from build123d import *

# Parameters (mm, degrees)
SKETCH_1_R          = 15
SKETCH_1_R_2        = 1.45
SKETCH_1_R_3        = 1.5
EXTRUDE_1_DEPTH     = 13
SKETCH_2_R          = 1.45
SKETCH_2_R_2        = 1.5
EXTRUDE_2_DEPTH     = 7
SKETCH_3_R          = 1.45
CUT_EXTRUDE_1_DEPTH = 38.5
SKETCH_4_R          = 1.45
CUT_EXTRUDE_2_DEPTH = 38.5
SKETCH_5_R          = 1.45
CUT_EXTRUDE_3_DEPTH = 31
SKETCH_8_R          = 1.5
CUT_EXTRUDE_6_DEPTH = 38.5
CHAMFER_1_SIZE      = 1.55


with BuildPart() as part:
    # 草图1 → 凸台-拉伸1 (new body)
    with BuildSketch(Plane(origin=(0, 0, 0), x_dir=(1, 0, 0), z_dir=(0, 1, 0))):
        Circle(SKETCH_1_R)
        with Locations((0, 12)):
            Circle(SKETCH_1_R_2, mode=Mode.SUBTRACT)
        with Locations((-10.392304845, -6)):
            Circle(SKETCH_1_R_2, mode=Mode.SUBTRACT)
        with Locations((10.392304845, -6)):
            Circle(SKETCH_1_R_2, mode=Mode.SUBTRACT)
        with Locations((-11.258330249, 6.5)):
            Circle(SKETCH_1_R_3, mode=Mode.SUBTRACT)
        with Locations((0, -13)):
            Circle(SKETCH_1_R_3, mode=Mode.SUBTRACT)
        with Locations((11.258330249, 6.5)):
            Circle(SKETCH_1_R_3, mode=Mode.SUBTRACT)
    extrude(amount=EXTRUDE_1_DEPTH)

    # 草图2 → 凸台-拉伸2 (add)
    with BuildSketch(Plane(origin=(0, 13, 0), x_dir=(1, 0, 0), z_dir=(0, 1, 0))):
        Polygon((0, 17.320508076), (-15, 8.660254038), (-15, -8.660254038), (0, -17.320508076), (15, -8.660254038), (15, 8.660254038), align=None)
        with Locations((0, 12)):
            Circle(SKETCH_2_R, mode=Mode.SUBTRACT)
        with Locations((-11.258330249, 6.5)):
            Circle(SKETCH_2_R_2, mode=Mode.SUBTRACT)
        with Locations((11.258330249, 6.5)):
            Circle(SKETCH_2_R_2, mode=Mode.SUBTRACT)
        with Locations((-10.392304845, -6)):
            Circle(SKETCH_2_R, mode=Mode.SUBTRACT)
        with Locations((0, -13)):
            Circle(SKETCH_2_R_2, mode=Mode.SUBTRACT)
        with Locations((10.392304845, -6)):
            Circle(SKETCH_2_R, mode=Mode.SUBTRACT)
    extrude(amount=-EXTRUDE_2_DEPTH)

    # 草图3 → 切除-拉伸1 (cut, through all)
    with BuildSketch(Plane(origin=(7.5, 0, 12.990381057), x_dir=(0.866025404, 0, -0.5), z_dir=(0.5, 0, 0.866025404))):
        with Locations((0, 9.5)):
            Circle(SKETCH_3_R)
    extrude(amount=-CUT_EXTRUDE_1_DEPTH, mode=Mode.SUBTRACT)

    # 草图4 → 切除-拉伸2 (cut, through all)
    with BuildSketch(Plane(origin=(-7.5, 0, 12.990381057), x_dir=(0.866025404, 0, 0.5), z_dir=(-0.5, 0, 0.866025404))):
        with Locations((0, 9.5)):
            Circle(SKETCH_4_R)
    extrude(amount=-CUT_EXTRUDE_2_DEPTH, mode=Mode.SUBTRACT)

    # 草图5 → 切除-拉伸3 (cut, through all)
    with BuildSketch(Plane.ZY.offset(15)):
        with Locations((0, 9.5)):
            Circle(SKETCH_5_R)
    extrude(amount=-CUT_EXTRUDE_3_DEPTH, mode=Mode.SUBTRACT)

    # 草图8 → 切除-拉伸6 (cut, through all)
    with BuildSketch(Plane(origin=(-7.5, 0, -12.990381057), x_dir=(-0.866025404, 0, 0.5), z_dir=(-0.5, 0, -0.866025404))):
        with Locations((0, 9.5)):
            Circle(SKETCH_8_R)
    extrude(amount=-CUT_EXTRUDE_6_DEPTH, mode=Mode.SUBTRACT)

    # 倒角1
    chamfer_1_edges = [part.edges().sort_by_distance(p)[0] for p in [
        (8.942304845, 13, 6),
        (-1.45, 13, -12),
        (-11.842304845, 13, 6),
    ]]
    chamfer(chamfer_1_edges, length=CHAMFER_1_SIZE)


solid = part.part
Design review of the part built by this model. Coordinates are the model's own, in mm. A direction names the side the tool comes from. Give positions to 0.01 mm unless a question says otherwise; leave off trailing zeros. Answer as a JSON object with one key per item and string values. Group by question number.
1) For line 1 along X through (y, z) = (3.5, 6); line 2 along Z through (x, y) = (0, 5); line 3 along Y through (x, z) = (6.5, 11), list the stretches that pass through material, from the lowest coordinate up.
2) We need section A-A (y = 8.5). Count the separate pieces of the cut face and the enclosed holes in it, and give its area (3 significant figures).
3) Tool access review of faces 1 (the face through (0, 6, 15.5)), 2 (the face through (13, 6, 8)), 3 (the face through (7.59, 9.56, -1.45)): name each direction out of +Z, -Z, +X, -X, +Y, -Y from which nothing blocks a thin tool from reaching the whole face with its end or side.
4) Clearance check with flat-ended pins moving along their axes: pin 1 Ø4 at (x, z) = (-11.26, -6.5) entering from -Y; pin 2 Ø1 at (y, z) = (8.5, 10.5) entering from -X; pin 3 Ø5 at (x, y) = (8.5, 1.5) entering from +Z; pin 4 Ø1.5 at (x, z) = (10.5, 7) entering from +Y. State where each tip first meets the part, or that it passes through.
5) Mouldability with a two-part tool opening along X and no side actions: class faces 4 (the face through (-0.325, 6.409, 14.464)), 5 (the face through (-13.5, 6, -7.5)), 6 (the face through (0, 8, 0)), 7 (the face through (7.605, 11.105, -12.93)) as released by +X, released by -X, zero draft, split by the parting line, or undercut.
Answer key:
{
 "1": {"line 1": "x = -13.75 to -11.84, -8.94 to 8.94, 11.84 to 13.75", "line 2": "z = -15 to -13.45, -10.55 to 11.5, 14.5 to 15", "line 3": "y = 0 to 8.01, 10.99 to 13"},
 "2": {"separate pieces": "6", "enclosed holes": "6", "area": "557 mm²"},
 "3": {"face 1": "+Z, -Y", "face 2": "+Z, +X, -Y", "face 3": "+X, -X"},
 "4": {"pin 1": "stops at y = 0", "pin 2": "stops at x = -12.68", "pin 3": "stops at z = 13.75", "pin 4": "stops at y = 11.76"},
 "5": {"face 4": "undercut", "face 5": "zero draft", "face 6": "undercut", "face 7": "released by +X"}
}
